Autodesk Inventor part; units mm, degrees
ref_plane "YZ Plane" through (0, 0, 0) normal (1, 0, 0) x (0, 1, 0)
ref_plane "XZ Plane" through (0, 0, 0) normal (0, 1, 0) x (-1, 0, 0)
ref_plane "XY Plane" through (0, 0, 0) normal (0, 0, 1) x (1, 0, 0)
sketch "Szkic1" plane through (0, 0, 0) normal (0, 0, 1) x (1, 0, 0)
  line L0 (-9.6, 0) -> (1.6, 0) construction
  line L1 (0, -3.6196) -> (0, 21.7176) construction
  line L2 (0, 0) -> (-8, 0)
  line L3 (-8, 0) -> (-8, 14.098)
  line L4 (-8, 14.098) -> (0, 14.098)
  line L5 (0, 14.098) -> (0, 0)
  circle A0 centre (-4, 14.098) radius 4
  dimension "d1" = 8
  dimension "d2" = 14.098
extrude "Wyciągnięcie proste1" add sketch "Szkic1" along normal blind 2
hole "Otwór1" at (-4, 14.098, 0) direction (0, 0, 1) diameter 2 end through all
fillet "Zaokrąglenie1" radius 2 3 edges at (-4, 18.098, 0) (-8, 7.049, 0) (0, 7.049, 0)
properties part number "podpora"
For this review, take the finished solid that the model builds, in its own axes (mm). Give positions to 0.01 mm unless a question says otherwise; leave off trailing zeros. Order: outer loops, then holes, each group sorted by start corner. A loop starts at its lowest first (then second) coordinate and runs counter-clockwise, first axis right, second up.
1) Take a section at D-D (z = 0.4). Give the boundary of the cut face in (x, y), then the cut area to 3 significant figures.
2) The part is to be moulded in two halves that separate along Y. For faces 1 (the face through (-4, 8, 0)), 2 (the face through (-4.3, 15.05, 1.01)), 3 (the face through (-4, 0, 1)), say which applies: released by +Y, released by -Y, zero draft, split by the parting line, or undercut.
3) Insertion check: pin 1 (1.8 mm diameter, centred on x = -4, y = 14.098, fed in from +Z). The pin has a flat end and moves straight along its axis. Give the tip position at first contact, or say it passes through.
4) Wall thickness on line 1 (X direction, y = 14, z = 1.5); line 2 (Y direction, x = -4, z = 1.15); line 3 (Y direction, x = -4, z = 0.4): over which ranges is each line inside the solid? List them lowest first.
5) Take a section at C-C (z = 1.35). Give the boundary of the cut face in (x, y), then the cut area to 3 significant figures.
Derived:
1. outline: (-7.2, 0) - (-0.8, 0) - (-0.8, 14.1) arc R3.2 ccw to (-7.2, 14.1) - close; hole circle Ø2 at (-4, 14.1)
1. area: 103 mm2
2. face 1: zero draft
2. face 2: undercut
2. face 3: released by -Y
3. pin 1: passes through
4. line 1: x = -7.94 to -5, -3 to -0.06
4. line 2: y = 0 to 13.1, 15.1 to 17.91
4. line 3: y = 0 to 13.1, 15.1 to 17.3
5. outline: (-7.89, 0) - (-0.11, 0) - (-0.11, 14.1) arc R3.89 ccw to (-7.89, 14.1) - close; hole circle Ø2 at (-4, 14.1)
5. area: 130 mm2
